Here's how the part is built. I have some questions about the finished solid (model axes, mm). Face numbers are marked on the shaded views. Coordinates: 2 decimals unless noted, no trailing zeros. Write each loop counter-clockwise with the first axis right and the second up, starting at its lowest first coordinate (ties: lowest second). Pieces come first, ordered by that corner, then holes. Notation, with made-up numbers: (50.5, 7.25) -> (96.5, 7.25) arc R26 cw to (96.5, 23.25) -> close; hole circle Ø11 at (-11, -36). An arc over 180 degrees is marked (long way). Use a Markdown table: item, result. Add a question column.
Item 1: Imagine slicing it at D-D, the plane y = 64. Write out the boundary of the cut face in (x, z) (3 decimals).
Item 2: Will these pins go through, and if not, where does the flat tip stop? pin 1 Ø17 at (x, y) = (-67, 90) entering from -Z; pin 2 Ø4 at (x, y) = (-70, -96.65) entering from +Z; pin 3 Ø0.5 at (y, z) = (94.5, -8.5) entering from +X (3 decimals); pin 4 Ø4 at (x, y) = (-64.5, -67) entering from -Z.
Item 3: If we mould it in two halves opening along Y, with no side actions, what happens to the marked faces 1 and 2? For each: pulls with the +Y half, pulls with the -Y half, needs draft (parallel to the pull), parting line crosses it, or undercut.
Item 4: If I drill on line 1 along X through (y, z) = (0, -6.8); line 2 along X through (y, z) = (90, -7.6); line 3 along Y through (x, z) = (80, -7.65), over which ranges is the centre line in solid material (lowest first)? Write a range as from..to.
Item 5: Imagine slicing it at A-A, the plane x = 80. Write out the boundary of the cut face in (y, z).
Item 6: Imagine slicing it at C-C, the plane x = 25.5. Write out the boundary of the cut face in (y, z), and give its area (3 significant figures).
Item 7: Imagine slicing it at B-B, the plane y = 90. Write out the boundary of the cut face in (x, z) (3 decimals).
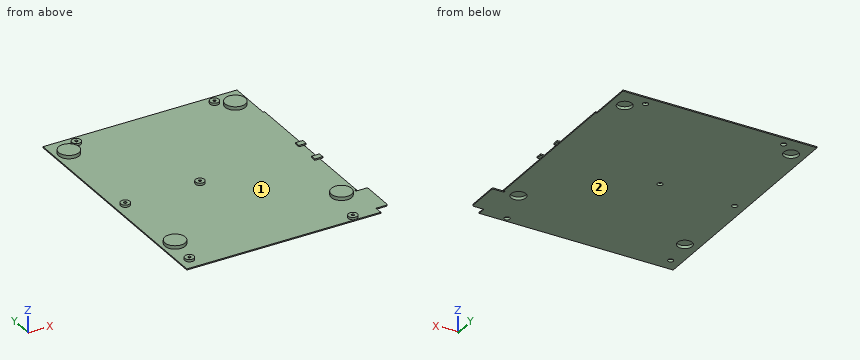
```python
from build123d import *

# Parameters (mm, degrees)
PAD010_DEPTH    = 1
SKETCH046_R     = 9
PAD011_DEPTH    = 4
SKETCH047_R     = 6.5
POCKET029_DEPTH = 2.6
SKETCH050_R     = 4
PAD012_DEPTH    = 3
SKETCH051_R     = 2.4
POCKET031_DEPTH = 2
SKETCH052_R     = 1.25
POCKET032_DEPTH = 5
SKETCH059_W     = 7
SKETCH059_H     = 5
SKETCH059_W_2   = 6.41159
PAD013_DEPTH    = 1.2


with BuildPart() as part:
    # Sketch044 (on DatumPlane) → Pad010 (new body)
    with BuildSketch(Plane(origin=(0, 0, -9), x_dir=(1, 0, 0), z_dir=(0, 0, -1))):
        with BuildLine():
            Line((-79.145, 108.35), (-79.145, -108.35))
            Line((-79.145, -108.35), (92.255, -108.35))
            Line((92.255, -108.35), (92.255, -69.206169))
            Line((93.544304, -69.206169), (92.255, -69.206169))
            Line((93.544304, 69.259346), (93.544304, -69.206169))
            Line((92.24646, 69.259346), (93.544304, 69.259346))
            Line((92.24646, 69.259346), (92.24646, 70.93325))
            Line((92.24646, 70.93325), (101.038879, 70.93325))
            ThreePointArc((101.038879, 70.93325), (102.099539, 71.37259), (102.538879, 72.43325))
            Line((102.538879, 72.43325), (102.538879, 99.723724))
            ThreePointArc((102.538879, 99.723724), (102.099539, 100.784384), (101.038879, 101.223724))
            Line((101.038879, 101.223724), (92.24646, 101.223724))
            Line((92.24646, 101.223724), (92.24646, 108.35))
            Line((92.24646, 108.35), (-79.145, 108.35))
        make_face()
    extrude(amount=-PAD010_DEPTH)

    # Sketch046 (on DatumPlane) → Pad011 (join)
    with BuildSketch(Plane(origin=(0, 0, -9), x_dir=(1, 0, 0), z_dir=(0, 0, -1))):
        with Locations((-67.0755, 70)):
            Circle(SKETCH046_R)
        with Locations((80, 70)):
            Circle(SKETCH046_R)
        with Locations((80, -90)):
            Circle(SKETCH046_R)
        with Locations((-67, -90)):
            Circle(SKETCH046_R)
    extrude(amount=-PAD011_DEPTH)

    # Sketch047 (on DatumPlane) → Pocket029 (cut)
    with BuildSketch(Plane(origin=(0, 0, -9), x_dir=(1, 0, 0), z_dir=(0, 0, -1))):
        with Locations((-67, 70)):
            Circle(SKETCH047_R)
        with Locations((80, 70)):
            Circle(SKETCH047_R)
        with Locations((80, -90)):
            Circle(SKETCH047_R)
        with Locations((-67, -90)):
            Circle(SKETCH047_R)
    extrude(amount=-POCKET029_DEPTH, mode=Mode.SUBTRACT)

    # Sketch050 (on DatumPlane) → Pad012 (join)
    with BuildSketch(Plane(origin=(0, 0, -9), x_dir=(1, 0, 0), z_dir=(0, 0, -1))):
        with Locations((-70, 0)):
            Circle(SKETCH050_R)
        with Locations((-70, 96.649681)):
            Circle(SKETCH050_R)
        with Locations((-4, 0)):
            Circle(SKETCH050_R)
        with Locations((67.474617, -100)):
            Circle(SKETCH050_R)
        with Locations((-54.612518, -100)):
            Circle(SKETCH050_R)
        with Locations((70, 104.126282)):
            Circle(SKETCH050_R)
    extrude(amount=-PAD012_DEPTH)

    # Sketch051 (on DatumPlane) → Pocket031 (cut)
    with BuildSketch(Plane(origin=(0, 0, -9), x_dir=(1, 0, 0), z_dir=(0, 0, -1))):
        with Locations((-70, 0)):
            Circle(SKETCH051_R)
        with Locations((-4, 0)):
            Circle(SKETCH051_R)
        with Locations((67.474617, -100)):
            Circle(SKETCH051_R)
        with Locations((-54.612518, -100)):
            Circle(SKETCH051_R)
        with Locations((-70, 96.649681)):
            Circle(SKETCH051_R)
        with Locations((70, 104.185745)):
            Circle(SKETCH051_R)
    extrude(amount=-POCKET031_DEPTH, mode=Mode.SUBTRACT)

    # Sketch052 (on DatumPlane) → Pocket032 (cut)
    with BuildSketch(Plane(origin=(0, 0, -9), x_dir=(1, 0, 0), z_dir=(0, 0, -1))):
        with Locations((-54.612518, -100)):
            Circle(SKETCH052_R)
        with Locations((67.474617, -100)):
            Circle(SKETCH052_R)
        with Locations((-4, 0)):
            Circle(SKETCH052_R)
        with Locations((-70, 0)):
            Circle(SKETCH052_R)
        with Locations((70.000001, 104.129997)):
            Circle(SKETCH052_R)
        with Locations((-70, 96.649681)):
            Circle(SKETCH052_R)
    extrude(amount=-POCKET032_DEPTH, mode=Mode.SUBTRACT)

    # Sketch059 (on DatumPlane) → Pad013 (join)
    with BuildSketch(Plane(origin=(0, 0, -8), x_dir=(1, 0, 0), z_dir=(0, 0, -1))):
        with Locations((92.5, 12)):
            Rectangle(SKETCH059_W, SKETCH059_H)
        with Locations((92.205795, -12)):
            Rectangle(SKETCH059_W_2, SKETCH059_H)
    extrude(amount=-PAD013_DEPTH)


solid = part.part
```
Ans:
| question | item | result |
|---|---|---|
| 1 | outline | (-79.145, -9) -> (93.544, -9) -> (93.544, -8) -> (-79.145, -8) -> close |
| 2 | pin 1 | stops at z = -9 |
| 2 | pin 2 | stops at z = -6 |
| 2 | pin 3 | stops at x = 92.255 |
| 2 | pin 4 | stops at z = -6.4 |
| 3 | face 1 | undercut |
| 3 | face 2 | needs draft |
| 4 | line 1 | x = -74..-71.25, -68.75..-66, -8..-5.25, -2.75..0 |
| 4 | line 2 | x = -76..-73.5, -60.5..-58, 71..73.5, 86.5..89 |
| 4 | line 3 | y = -79..-76.5, -63.5..-61, 81..83.5, 96.5..99 |
| 5 | outline | (-108.35, -9) -> (-76.5, -9) -> (-76.5, -6.4) -> (-63.5, -6.4) -> (-63.5, -9) -> (83.5, -9) -> (83.5, -6.4) -> (96.5, -6.4) -> (96.5, -9) -> (108.35, -9) -> (108.35, -8) -> (99, -8) -> (99, -5) -> (81, -5) -> (81, -8) -> (-61, -8) -> (-61, -5) -> (-79, -5) -> (-79, -8) -> (-108.35, -8) -> close |
| 6 | outline | (-108.35, -9) -> (108.35, -9) -> (108.35, -8) -> (-108.35, -8) -> close |
| 6 | area | 217 mm^2 |
| 7 | outline | (-79.145, -9) -> (-73.5, -9) -> (-73.5, -6.4) -> (-60.5, -6.4) -> (-60.5, -9) -> (73.5, -9) -> (73.5, -6.4) -> (86.5, -6.4) -> (86.5, -9) -> (92.255, -9) -> (92.255, -8) -> (89, -8) -> (89, -5) -> (71, -5) -> (71, -8) -> (-58, -8) -> (-58, -5) -> (-76, -5) -> (-76, -8) -> (-79.145, -8) -> close |
